Input: part model. Units: mm. Frame: model coordinates. Face numbers are marked on the shaded views. A direction names the side the tool comes from. Give positions to 0.01 mm unless a question says otherwise; leave off trailing zeros. Loops run counter-clockwise (first coordinate to the right, second up) from the corner with the lowest first, then second, coordinate; pieces in that order, holes last. Notation, with made-up numbers: M 54.5,13.25 L 91.5,13.25 A19 ccw 91.5,18.25 Z; hole C 2.25,67 d4. An arc over 180 degrees is marked long. Answer as a JSON object with one key per item and string values. Group by question number.
```python
from build123d import *

# Parameters (mm, degrees)
SKETCH1_W           = 25
SKETCH1_H           = 14.7
BOSS_EXTRUDE1_DEPTH = 2
FILLET1_R           = 6
BOSS_EXTRUDE6_DEPTH = 2
SKETCH5_R           = 0.7
BOSS_EXTRUDE7_DEPTH = 1.5


with BuildPart() as part:
    # Sketch1 → Boss-Extrude1 (new body)
    with BuildSketch(Plane(origin=(0, 0, 0), x_dir=(1, 0, 0), z_dir=(0, 1, 0))):
        Rectangle(SKETCH1_W, SKETCH1_H)
    extrude(amount=BOSS_EXTRUDE1_DEPTH)

    # Fillet1
    fillet1_edges = [part.edges().sort_by_distance(p)[0] for p in [
        (12.5, 1, 7.35),
        (-12.5, 1, 7.35),
        (-12.5, 1, -7.35),
        (12.5, 1, -7.35),
    ]]
    fillet(fillet1_edges, radius=FILLET1_R)

    # Sketch3 → Boss-Extrude6 (add)
    with BuildSketch(Plane(origin=(0, 0, -7.35), x_dir=(-1, 0, 0), z_dir=(0, 0, -1))):
        with BuildLine():
            Line((-1.5, 0), (-1.5, -3))
            ThreePointArc((-1.5, -3), (-1.207106781, -3.707106781), (-0.5, -4))
            Line((-0.5, -4), (0.5, -4))
            ThreePointArc((0.5, -4), (1.207106781, -3.707106781), (1.5, -3))
            Line((1.5, -3), (1.5, 0))
            Line((1.5, 0), (-1.5, 0))
        make_face()
    boss_extrude6 = extrude(amount=-BOSS_EXTRUDE6_DEPTH)

    # Sketch5 → Boss-Extrude7 (add)
    with BuildSketch(Plane(origin=(0, 0, -7.35), x_dir=(-1, 0, 0), z_dir=(0, 0, -1))):
        with Locations(Location((0, -2.1, 0), (0, 0, 180))):  # turned: the seam where the file's is
            Circle(SKETCH5_R)
    boss_extrude7 = extrude(amount=BOSS_EXTRUDE7_DEPTH)

    # Mirror3: Boss-Extrude6, Boss-Extrude7 across plane
    add(boss_extrude6.mirror(Plane.XY))
    add(boss_extrude7.mirror(Plane.XY))


solid = part.part
```
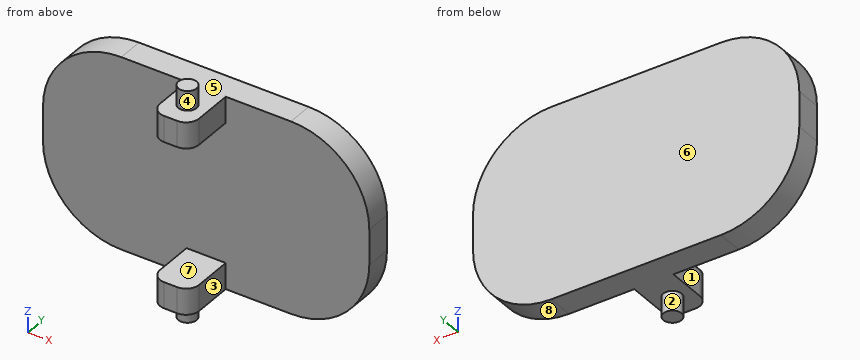
1. Section A-A (y = -2.1). Output: boundary loops of the cut face in (x, z).
2. First-contact query: P1, Ø0.6, axis at y = -1, z = -6.5, coming from the +X side; P2, Ø3, axis at y = -0.5, z = 6.5, coming from the +X side; P3, Ø0.6, axis at y = -1, z = 6, coming from the -X side. Flat tips, straight axial feed; report the tip coordinate or a pass-through.
3. Material intervals for L1, parallel to Z at x = 0.5, y = -0.6; L2, parallel to X at y = -2.3, z = -5.75; L3, parallel to Y at x = -6.75, z = -4, sorted ascending.
4. Reachability of the marked faces 1, 2, 3 and 4 from +Z, -Z, +X, -X, +Y, -Y: full face, straight path, thin tool, end or side. Return the list, or none.
5. Section C-C (z = 5.75). Output: boundary loops of the cut face in (x, y).
6. Mould query, pull axis Z, two halves, no side actions, for the marked faces 5, 6, 7 and 8. Classes: pulls with the +Z half, pulls with the -Z half, needs draft (parallel to the pull), parting line crosses it, or undercut.
7. Section B-B (x = 0). Output: boundary loops of the cut face in (y, z), then the cut area to 3 significant figures.
8. Section D-D (y = 0.6). Output: boundary loops of the cut face in (x, z), then the cut area to 3 significant figures.
Geometry results:
{
 "1": {"outline": "M -1.5,-7.35 L -0.7,-7.35 L -0.7,-8.85 L 0.7,-8.85 L 0.7,-7.35 L 1.5,-7.35 L 1.5,-5.35 L -1.5,-5.35 Z; M -1.5,5.35 L 1.5,5.35 L 1.5,7.35 L 0.7,7.35 L 0.7,8.85 L -0.7,8.85 L -0.7,7.35 L -1.5,7.35 Z"},
 "2": {"P1": "x = 1.5", "P2": "x = 11.2", "P3": "x = -1.5"},
 "3": {"L1": "-7.35 to -5.35, 5.35 to 7.35", "L2": "-1.5 to 1.5", "L3": "0 to 2"},
 "4": {"face 1": "+Z, -Z, -X, -Y", "face 2": "-Z", "face 3": "+Z, -Z, +X, -Y", "face 4": "+Z"},
 "5": {"outline": "M -10.58,0 L -1.5,0 L -1.5,-3 A1 ccw -0.5,-4 L 0.5,-4 A1 ccw 1.5,-3 L 1.5,0 L 10.58,0 L 10.58,2 L -10.58,2 Z"},
 "6": {"face 5": "pulls with the +Z half", "face 6": "needs draft", "face 7": "undercut", "face 8": "pulls with the -Z half"},
 "7": {"outline": "M -4,-7.35 L -2.8,-7.35 L -2.8,-8.85 L -1.4,-8.85 L -1.4,-7.35 L 2,-7.35 L 2,7.35 L -1.4,7.35 L -1.4,8.85 L -2.8,8.85 L -2.8,7.35 L -4,7.35 L -4,5.35 L 0,5.35 L 0,-5.35 L -4,-5.35 Z", "area": "49.6 mm2"},
 "8": {"outline": "M -12.5,-1.35 A6 ccw -6.5,-7.35 L 6.5,-7.35 A6 ccw 12.5,-1.35 L 12.5,1.35 A6 ccw 6.5,7.35 L -6.5,7.35 A6 ccw -12.5,1.35 Z", "area": "337 mm2"}
}
